Source: CAD feature listing. Evaluate the final solid. Frame: model axes, mm. Round coordinates to 2 decimals unless told otherwise and drop trailing zeros. Loops run counter-clockwise (first coordinate to the right, second up) from the corner with the lowest first, then second, coordinate; pieces in that order, holes last.
Item 1: Section query B-B on y = 17.5. Return loops of the section in (x, z).
Item 2: Ray query, L1, parallel to X at y = 40, z = 0; L2, parallel to Z at x = -0.1, y = 36; L3, parallel to Z at x = 1, y = 50.5. Return the intervals inside material, ascending.
Item 3: Section query A-A on x = 0. Return loops of the section in (y, z), then the cut area to 3 significant figures.
Item 4: First-contact query: P1, Ø1, axis at y = 32, z = 0.5, coming from the -X side; P2, Ø2, axis at y = 23.5, z = -1.5, coming from the -X side; P3, Ø1.5, axis at x = 0, z = 0, coming from the +Y side. Flat tips, straight axial feed; report the tip coordinate or a pass-through.
```python
from build123d import *

# Parameters (mm, degrees)
SKETCH_1_R      = 1.5
EXTRUDE_1_DEPTH = 60
FILLET_1_R      = 0.3


with BuildPart() as part:
    # 草图1 → 凸台-拉伸1 (new body)
    with BuildSketch(Plane(origin=(0, 0, 0), x_dir=(1, 0, 0), z_dir=(0, 1, 0))):
        Polygon((2.713546265, 0), (1.356773133, 2.35), (-1.356773133, 2.35), (-2.713546265, 0), (-1.356773133, -2.35), (1.356773133, -2.35), align=None)
        with Locations(Location((0, 0, 0), (0, 0, 270))):
            Circle(SKETCH_1_R, mode=Mode.SUBTRACT)
    extrude(amount=EXTRUDE_1_DEPTH)

    # 圆角1
    fillet_1_edges = [part.edges().sort_by_distance(p)[0] for p in [
        (0, 60, -2.35),
        (1.356773133, 30, 2.35),
        (-1.356773133, 30, 2.35),
        (-2.713546265, 30, 0),
        (-1.356773133, 30, -2.35),
        (1.356773133, 30, -2.35),
        (2.713546265, 30, 0),
        (-2.035159699, 60, -1.175),
        (-2.035159699, 60, 1.175),
        (0, 60, 2.35),
        (2.035159699, 60, 1.175),
        (0, 0, 2.35),
        (-2.035159699, 0, 1.175),
        (-2.035159699, 0, -1.175),
        (2.035159699, 60, -1.175),
        (0, 0, -2.35),
        (2.035159699, 0, -1.175),
        (2.035159699, 0, 1.175),
    ]]
    fillet(fillet_1_edges, radius=FILLET_1_R)


solid = part.part
```
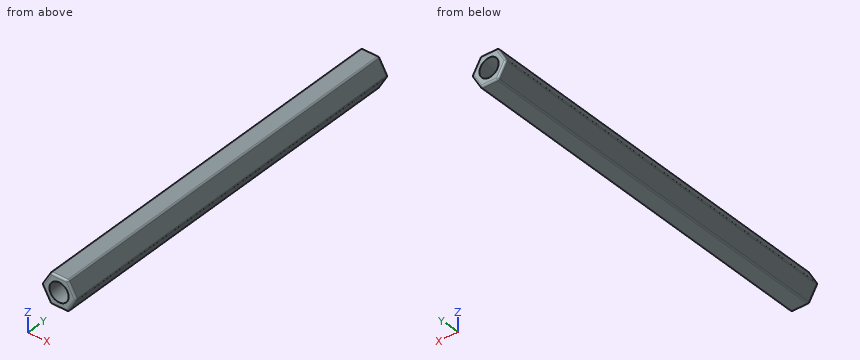
Data:
1. outline: (-2.63, -0.15) - (-1.44, -2.2) arc R0.3 ccw to (-1.18, -2.35) - (1.18, -2.35) arc R0.3 ccw to (1.44, -2.2) - (2.63, -0.15) arc R0.3 ccw to (2.63, 0.15) - (1.44, 2.2) arc R0.3 ccw to (1.18, 2.35) - (-1.18, 2.35) arc R0.3 ccw to (-1.44, 2.2) - (-2.63, 0.15) arc R0.3 ccw to start; hole circle Ø3 at (0, 0)
2. L1: x = -2.67 to -1.5, 1.5 to 2.67
2. L2: z = -2.35 to -1.5, 1.5 to 2.35
2. L3: z = -2.35 to -1.12, 1.12 to 2.35
3. outline: (0, -2.05) arc R0.3 ccw to (0.3, -2.35) - (59.7, -2.35) arc R0.3 ccw to (60, -2.05) - (60, -1.5) - (0, -1.5) - close; (0, 1.5) - (60, 1.5) - (60, 2.05) arc R0.3 ccw to (59.7, 2.35) - (0.3, 2.35) arc R0.3 ccw to (0, 2.05) - close
3. area: 102 mm2
4. P1: stops at x = -2.67
4. P2: stops at x = -2.42
4. P3: passes through
